from build123d import *

# Parameters (mm, degrees)
SKETCH_1_W          = 109.5
SKETCH_1_H          = 45
EXTRUDE_1_DEPTH     = 3
SKETCH_2_R          = 1.25
CUT_EXTRUDE_1_DEPTH = 10
SKETCH_3_R          = 1.65
CUT_EXTRUDE_2_DEPTH = 10
FILLET_1_R          = 3
CUT_EXTRUDE_3_DEPTH = 4


with BuildPart() as part:
    # 草图1 → 凸台-拉伸1 (new body)
    with BuildSketch(Plane(origin=(0, 0, 0), x_dir=(1, 0, 0), z_dir=(0, 1, 0))):
        Rectangle(SKETCH_1_W, SKETCH_1_H)
    extrude(amount=EXTRUDE_1_DEPTH)

    # 草图2 → 切除-拉伸1 (cut)
    with BuildSketch(Plane(origin=(0, 3, 0), x_dir=(1, 0, 0), z_dir=(0, 1, 0))):
        with Locations((9, 18.5)):
            Circle(SKETCH_2_R)
        with Locations((-9, 18.5)):
            Circle(SKETCH_2_R)
    extrude(amount=-CUT_EXTRUDE_1_DEPTH, mode=Mode.SUBTRACT)

    # 草图3 → 切除-拉伸2 (cut)
    with BuildSketch(Plane(origin=(0, 3, 0), x_dir=(1, 0, 0), z_dir=(0, 1, 0))):
        with Locations((-46.75, 7.5)):
            Circle(SKETCH_3_R)
        with Locations((46.75, 7.5)):
            Circle(SKETCH_3_R)
    extrude(amount=-CUT_EXTRUDE_2_DEPTH, mode=Mode.SUBTRACT)

    # 圆角1
    fillet_1_edges = [part.edges().sort_by_distance(p)[0] for p in [
        (54.75, 1.5, 22.5),
        (-54.75, 1.5, 22.5),
        (-54.75, 1.5, -22.5),
        (54.75, 1.5, -22.5),
    ]]
    fillet(fillet_1_edges, radius=FILLET_1_R)

    # 草图4 → 切除-拉伸3 (cut, through all)
    with BuildSketch(Plane(origin=(0, 3, 0), x_dir=(1, 0, 0), z_dir=(0, 1, 0))):
        with BuildLine():
            Line((-38.45, 15), (-38.45, -15))
            ThreePointArc((-38.45, -15), (-39.75, -16.3), (-41.05, -15))
            Line((-41.05, -15), (-41.05, 15))
            ThreePointArc((-41.05, 15), (-39.75, 16.3), (-38.45, 15))
        make_face()
        with BuildLine():
            Line((-32.45, 15), (-32.45, -15))
            ThreePointArc((-32.45, -15), (-33.75, -16.3), (-35.05, -15))
            Line((-35.05, -15), (-35.05, 15))
            ThreePointArc((-35.05, 15), (-33.75, 16.3), (-32.45, 15))
        make_face()
        with BuildLine():
            Line((-26.45, 15), (-26.45, -15))
            ThreePointArc((-26.45, -15), (-27.75, -16.3), (-29.05, -15))
            Line((-29.05, -15), (-29.05, 15))
            ThreePointArc((-29.05, 15), (-27.75, 16.3), (-26.45, 15))
        make_face()
        with BuildLine():
            Line((-20.45, 15), (-20.45, -15))
            ThreePointArc((-20.45, -15), (-21.75, -16.3), (-23.05, -15))
            Line((-23.05, -15), (-23.05, 15))
            ThreePointArc((-23.05, 15), (-21.75, 16.3), (-20.45, 15))
        make_face()
        with BuildLine():
            Line((-14.45, 15), (-14.45, -15))
            ThreePointArc((-14.45, -15), (-15.75, -16.3), (-17.05, -15))
            Line((-17.05, -15), (-17.05, 15))
            ThreePointArc((-17.05, 15), (-15.75, 16.3), (-14.45, 15))
        make_face()
        with BuildLine():
            Line((-8.45, 15), (-8.45, -15))
            ThreePointArc((-8.45, -15), (-9.75, -16.3), (-11.05, -15))
            Line((-11.05, -15), (-11.05, 15))
            ThreePointArc((-11.05, 15), (-9.75, 16.3), (-8.45, 15))
        make_face()
        with BuildLine():
            Line((-2.45, 15), (-2.45, -15))
            ThreePointArc((-2.45, -15), (-3.75, -16.3), (-5.05, -15))
            Line((-5.05, -15), (-5.05, 15))
            ThreePointArc((-5.05, 15), (-3.75, 16.3), (-2.45, 15))
        make_face()
        with BuildLine():
            Line((3.55, 15), (3.55, -15))
            ThreePointArc((3.55, -15), (2.25, -16.3), (0.95, -15))
            Line((0.95, -15), (0.95, 15))
            ThreePointArc((0.95, 15), (2.25, 16.3), (3.55, 15))
        make_face()
        with BuildLine():
            Line((9.55, 15), (9.55, -15))
            ThreePointArc((9.55, -15), (8.25, -16.3), (6.95, -15))
            Line((6.95, -15), (6.95, 15))
            ThreePointArc((6.95, 15), (8.25, 16.3), (9.55, 15))
        make_face()
        with BuildLine():
            Line((15.55, 15), (15.55, -15))
            ThreePointArc((15.55, -15), (14.25, -16.3), (12.95, -15))
            Line((12.95, -15), (12.95, 15))
            ThreePointArc((12.95, 15), (14.25, 16.3), (15.55, 15))
        make_face()
        with BuildLine():
            Line((21.55, 15), (21.55, -15))
            ThreePointArc((21.55, -15), (20.25, -16.3), (18.95, -15))
            Line((18.95, -15), (18.95, 15))
            ThreePointArc((18.95, 15), (20.25, 16.3), (21.55, 15))
        make_face()
        with BuildLine():
            Line((27.55, 15), (27.55, -15))
            ThreePointArc((27.55, -15), (26.25, -16.3), (24.95, -15))
            Line((24.95, -15), (24.95, 15))
            ThreePointArc((24.95, 15), (26.25, 16.3), (27.55, 15))
        make_face()
        with BuildLine():
            Line((33.55, 15), (33.55, -15))
            ThreePointArc((33.55, -15), (32.25, -16.3), (30.95, -15))
            Line((30.95, -15), (30.95, 15))
            ThreePointArc((30.95, 15), (32.25, 16.3), (33.55, 15))
        make_face()
        with BuildLine():
            Line((39.55, 15), (39.55, -15))
            ThreePointArc((39.55, -15), (38.25, -16.3), (36.95, -15))
            Line((36.95, -15), (36.95, 15))
            ThreePointArc((36.95, 15), (38.25, 16.3), (39.55, 15))
        make_face()
    extrude(amount=-CUT_EXTRUDE_3_DEPTH, mode=Mode.SUBTRACT)


solid = part.part
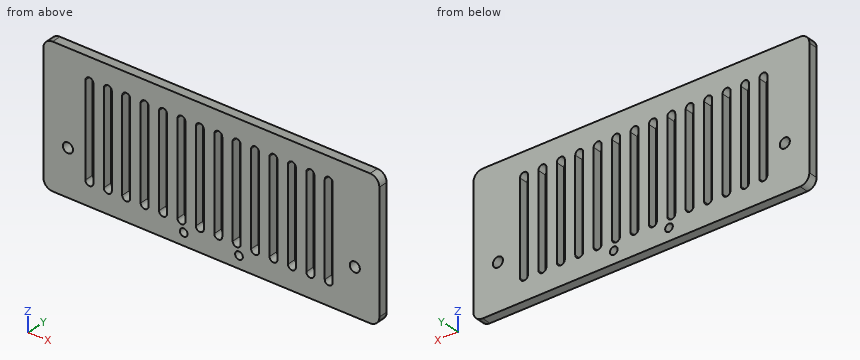
Source: CAD feature listing. Evaluate the final solid. Frame: model axes, mm. Round coordinates to 2 decimals unless told otherwise and drop trailing zeros. Loops run counter-clockwise (first coordinate to the right, second up) from the corner with the lowest first, then second, coordinate; pieces in that order, holes last. Notation, with made-up numbers: M 73,49 L 97,49 A33 ccw 97,86 Z; hole C 74,54.5 d11. An arc over 180 degrees is marked long. Return JSON: item names as keys, results as strings. Group by question number.
1. Section query C-C on y = 0.55. State how many separate pieces and enclosed holes the cut face has, and give its area (3 significant figures).
2. Section query A-A on x = -39.75. Output: boundary loops of the cut face in (y, z), and give its area (3 significant figures).
3. Section query B-B on z = -18.5. Output: boundary loops of the cut face in (x, y).
4. Material intervals for line 1 along X through (y, z) = (1.3, -18.5); line 2 along Z through (x, y) = (-39.5, 1.4); line 3 along Z through (x, y) = (46.75, 2.1), sorted ascending. Write a range as from..to.
Checks:
{
 "1": {"separate pieces": "1", "enclosed holes": "18", "area": "3,730 mm²"},
 "2": {"outline": "M 0,-22.5 L 3,-22.5 L 3,-16.3 L 0,-16.3 Z; M 0,16.3 L 3,16.3 L 3,22.5 L 0,22.5 Z", "area": "37.2 mm²"},
 "3": {"outline": "M -54.75,0 L -10.25,0 L -10.25,3 L -54.75,3 Z; M -7.75,0 L 7.75,0 L 7.75,3 L -7.75,3 Z; M 10.25,0 L 54.75,0 L 54.75,3 L 10.25,3 Z"},
 "4": {"line 1": "x = -54.75..-10.25, -7.75..7.75, 10.25..54.75", "line 2": "z = -22.5..-16.28, 16.28..22.5", "line 3": "z = -22.5..-9.15, -5.85..22.5"}
}
